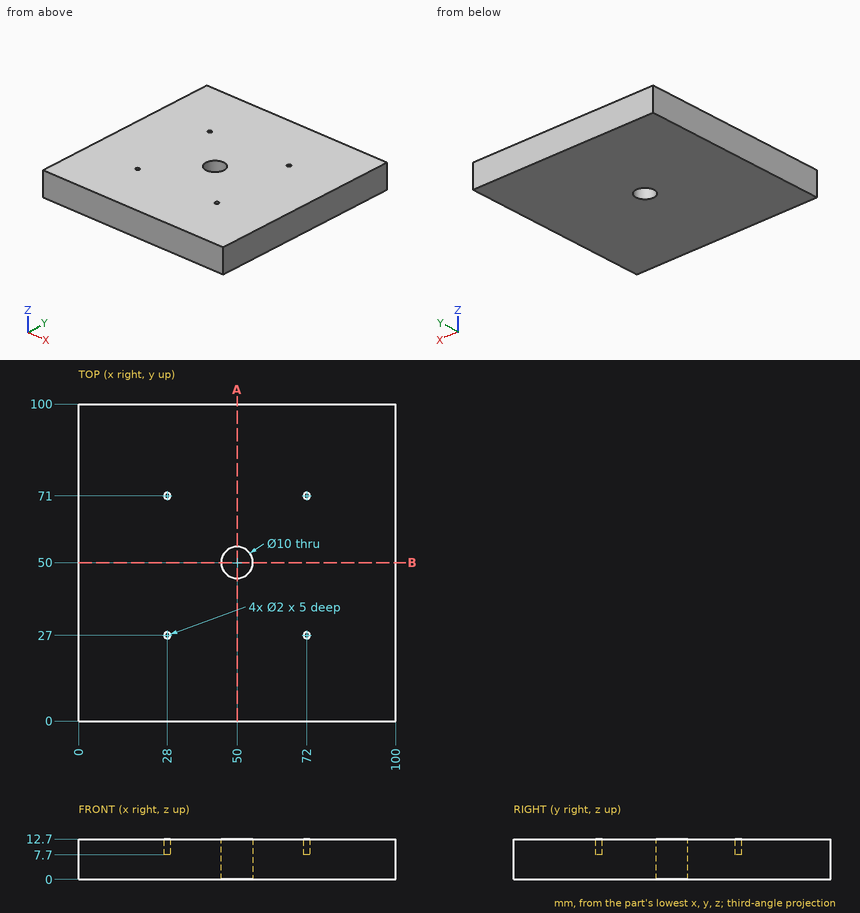
Verification items for this drawing (mm, ordinates from the low corner). Coordinates: 2 decimals unless noted, no trailing zeros. Loops run counter-clockwise (first coordinate to the right, second up) from the corner with the lowest first, then second, coordinate; pieces in that order, holes last. Notation, with made-up numbers: (47.25, 72.5) - (98.25, 72.5) arc R23 ccw to (98.25, 92.5) - close; hole circle Ø3 at (46, 49.5). An arc over 180 degrees is marked (long way). Answer as a JSON object with one key per item and string values.
(1) Go/stop test with flat-tipped pins: pin 1 Ø12 at (x, y) = (51, 61.5) entering from -Z; pin 2 Ø0.6 at (x, y) = (27.5, 27) entering from +Z. Record where each tip stops, or that it passes through.
Response:
{"pin 1": "stops at z = 0", "pin 2": "stops at z = 7.7"}
(2) Cross-section at A-A, the plane x = 50. Record the boundary of the cut face in (y, z), then the cut area to 3 significant figures.
Response:
{"outline": "(0, 0) - (45, 0) - (45, 12.7) - (0, 12.7) - close; (55, 0) - (100, 0) - (100, 12.7) - (55, 12.7) - close", "area": "1,140 mm²"}
(3) Scan lines: line 1 along Y through (x, z) = (28, 8.9); line 2 along X through (y, z) = (71, 9.95); line 3 along Y through (x, z) = (51, 2.5). Record each from-to range of solid material in increasing order.
Response:
{"line 1": "y = 0 to 26, 28 to 70, 72 to 100", "line 2": "x = 0 to 27, 29 to 71, 73 to 100", "line 3": "y = 0 to 45.1, 54.9 to 100"}
